```python
from build123d import *

# Parameters (mm, degrees)
EXTRUDE_1_DEPTH    = 2.5
HOLE_WIZARD_M3_1_D = 2.5
CHAMFER_1_SIZE     = 1


with BuildPart() as part:
    # 草图1 → 凸台-拉伸1 (new, symmetric)
    with BuildSketch(Plane.XY):
        Polygon((-5, -4.5), (5, -4.5), (5, 0), (10, 0), (10, -8.5), (-10, -8.5), (-10, 0), (-5, 0), align=None)
    extrude(amount=EXTRUDE_1_DEPTH, both=True)

    # M3 螺纹孔1 (through all)
    with Locations(Plane(origin=(0, -8.5, 0), x_dir=(-1, 0, 0), z_dir=(0, -1, 0))):
        with Locations((7.5, 0), (-7.5, 0)):
            Hole(HOLE_WIZARD_M3_1_D / 2)

    # 倒角1
    chamfer_1_edges = [part.edges().sort_by_distance(p)[0] for p in [
        (10, -8.5, 0),
        (-10, -8.5, 0),
        (-5, -4.5, 0),
        (5, -4.5, 0),
    ]]
    chamfer(chamfer_1_edges, length=CHAMFER_1_SIZE)


solid = part.part
```
Check sheet for the modelled part. Datum: model origin and axes. Units: mm. A direction names the side the tool comes from. Round coordinates to 2 decimals unless told otherwise and drop trailing zeros. Loops run counter-clockwise (first coordinate to the right, second up) from the corner with the lowest first, then second, coordinate; pieces in that order, holes last. Notation, with made-up numbers: M 16.5,-5 L 28.5,-5 A15 cw 28.5,10 Z; hole C -7,1 d2. An arc over 180 degrees is marked long. Answer as a JSON object with one key per item and string values.
1. Scan lines: line 1 (Z direction, x = 7.5, y = -3.5); line 2 (X direction, y = -4.25, z = 0.4); line 3 (X direction, y = -2.25, z = -0.15). Record each from-to range of solid material in increasing order.
Reply:
{"line 1": "z = -2.5 to -1.25, 1.25 to 2.5", "line 2": "x = -10 to -8.68, -6.32 to -4.25, 4.25 to 6.32, 8.68 to 10", "line 3": "x = -10 to -8.74, -6.26 to -5, 5 to 6.26, 8.74 to 10"}
2. Mould release check, pull along Z, two halves, no side actions. Record for faces 3 (the flat face through (-5, -2, 0)), 4 (the cylindrical face through (-8.75, -4.19, -0.05)), 5 (the flat face through (0, -5, -2.5)): pulls with the +Z half, pulls with the -Z half, needs draft (parallel to the pull), parting line crosses it, or undercut.
Reply:
{"face 3": "needs draft", "face 4": "undercut", "face 5": "pulls with the -Z half"}
3. Section check A-A (y = -3). Record the boundary of the cut face in (x, z).
Reply:
{"outline": "M -10,-2.5 L -5,-2.5 L -5,2.5 L -10,2.5 Z; M 5,-2.5 L 10,-2.5 L 10,2.5 L 5,2.5 Z; hole C -7.5,0 d2.5; hole C 7.5,0 d2.5"}
4. Access from +Z, -Z, +X, -X, +Y, -Y to the whole of each face (thin tool, end or side, straight path). Record for faces 1 (the flat face through (0, -5, 2.5)), 2 (the flat face through (-4.5, -4, 0)).
Reply:
{"face 1": "+Z, +X, -X, +Y, -Y", "face 2": "+Z, -Z, +Y"}
5. Section check C-C (x = -7.5). Record the boundary of the cut face in (y, z), plus the area to 4 significant figures.
Reply:
{"outline": "M -8.5,-2.5 L 0,-2.5 L 0,-1.25 L -8.5,-1.25 Z; M -8.5,1.25 L 0,1.25 L 0,2.5 L -8.5,2.5 Z", "area": "21.25 mm²"}
6. Section check D-D (y = -6.5). Record the boundary of the cut face in (x, z).
Reply:
{"outline": "M -10,-2.5 L 10,-2.5 L 10,2.5 L -10,2.5 Z; hole C -7.5,0 d2.5; hole C 7.5,0 d2.5"}
7. Section check B-B (z = 0). Record the boundary of the cut face in (x, y), plus the area to 3 significant figures.
Reply:
{"outline": "M -10,-7.5 L -9,-8.5 L -8.75,-8.5 L -8.75,0 L -10,0 Z; M -6.25,-8.5 L 6.25,-8.5 L 6.25,0 L 5,0 L 5,-3.5 L 4,-4.5 L -4,-4.5 L -5,-3.5 L -5,0 L -6.25,0 Z; M 8.75,-8.5 L 9,-8.5 L 10,-7.5 L 10,0 L 8.75,0 Z", "area": "82.5 mm²"}
8. Gauge pin test, flat end, axial feed: P1, Ø2.5, axis at x = -1.5, z = -0.5, coming from the +Y side. Record the tip position at first contact, or that the pin passes through.
Reply:
{"P1": "stops at y = -4.5"}
